Autodesk Inventor part; units mm, degrees
ref_plane "Work Plane1" through (22.86, 0, 0) normal (1, 0, 0) x (0, 1, 0)
ref_plane "XZ Plane" through (0, 0, 0) normal (0, 1, 0) x (-1, 0, 0)
ref_plane "XY Plane" through (0, 0, 0) normal (0, 0, 1) x (1, 0, 0)
sketch "Sketch1" plane through (0, 0, 0) normal (0, 1, 0) x (-1, 0, 0)
  circle A0 centre (0, 0) radius 22.86
  dimension "d0" = 45.72
extrude "Extrusion1" add sketch "Sketch1" along normal blind 99.06
sketch "Sketch2" plane through (0, 99.06, 0) normal (0, 1, 0) x (1, 0, 0)
  circle A0 centre (0, 0) radius 22.86
  circle A1 centre (0, -22.86) radius 9.906
  circle A2 centre (0, 22.86) radius 9.906
  dimension "d3" = 19.812
  dimension "d4" = 19.812
extrude "Extrusion2" add sketch "Sketch2" along normal blind 5.08
ref_plane "Work Plane1" through (22.86, 0, 0) normal (1, 0, 0) x (0, 1, 0)
properties part number "reducedLargeSyrginePlunger"
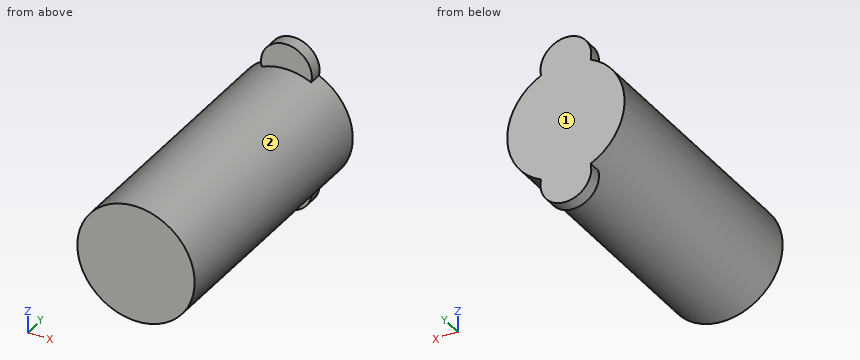
Input: part model. Units: mm. Frame: model coordinates. Face numbers are marked on the shaded views. A direction names the side the tool comes from. Coordinates: 2 decimals unless noted, no trailing zeros. Write each loop counter-clockwise with the first axis right and the second up, starting at its lowest first coordinate (ties: lowest second). Pieces come first, ordered by that corner, then holes.
1) Section C-C on y = 77.5. Output: boundary loops of the cut face in (x, z), and give its area (3 significant figures).
2) Section B-B on z = -7. Output: boundary loops of the cut face in (x, y), and give its area (3 significant figures).
3) Section D-D on z = 27.5. Output: boundary loops of the cut face in (x, y).
4) Pin query (flat end, axial travel): pin 1 Ø10 at (x, y) = (18, 62) entering from -Z; pin 2 Ø3 at (y, z) = (89.5, -5.5) entering from +X; pin 3 Ø1.5 at (x, y) = (14, 63) entering from -Z. Return the tip coordinate at first contact, or that it passes through.
5) Set-up query: the marked faces 1 and 2. Return all of +Z, -Z, +X, -X, +Y, -Y with unobstructed straight access to the full face (end or side cutting, diameter ignored); none if empty.
6) Material intervals for line 1 along Z through (x, y) = (1, 80); line 2 along Y through (x, z) = (-3, 27.5); line 3 along Z through (x, y) = (-17.5, 68), sorted ascending.
7) Section A-A on x = 0. Output: boundary loops of the cut face in (y, z), and give its area (3 significant figures).
Check result:
1. outline: circle Ø45.72 at (0, 0)
1. area: 1,640 mm2
2. outline: (-21.76, 0) - (21.76, 0) - (21.76, 104.14) - (-21.76, 104.14) - close
2. area: 4,530 mm2
3. outline: (-8.75, 99.06) - (8.75, 99.06) - (8.75, 104.14) - (-8.75, 104.14) - close
4. pin 1: stops at z = -18.8
4. pin 2: stops at x = 22.51
4. pin 3: stops at z = -18.63
5. face 1: +Z, -Z, +X, -X, +Y
5. face 2: -Y
6. line 1: z = -22.84 to 22.84
6. line 2: y = 99.06 to 104.14
6. line 3: z = -14.71 to 14.71
7. outline: (0, -22.86) - (99.06, -22.86) - (99.06, -32.77) - (104.14, -32.77) - (104.14, 32.77) - (99.06, 32.77) - (99.06, 22.86) - (0, 22.86) - close
7. area: 4,860 mm2
